CAD build for the part. Positions are in the model's coordinates, mm. Round coordinates to 2 decimals unless told otherwise and drop trailing zeros. Order: outer loops, then holes, each group sorted by start corner. A loop starts at its lowest first (then second) coordinate and runs counter-clockwise, first axis right, second up. Notation, with made-up numbers: (27, 26.25) -> (48, 26.25) arc R29 ccw to (48, 55.25) -> close; hole circle Ø9 at (84.25, -36). An arc over 180 degrees is marked (long way). Answer as CSV lines item,"result". Start each with the question number.
from build123d import *

# Parameters (mm, degrees)
SKETCH004_R          = 1.687519
PAD003_DEPTH         = 2
SKETCH003_R          = 1.746092
PAD002_DEPTH         = 2
FUSION001_ROLL_ANGLE = 90


with BuildPart() as base_and_horizontal_holder001:
    # Sketch004 → Pad003 (new body)
    with BuildSketch(Plane.XZ.offset(1.2525)):
        with BuildLine():
            Line((10.979984, 0), (69.999984, 0))
            Line((69.999984, 0), (69.999984, -21.282469))
            ThreePointArc((66.378106, -24.904346), (68.939161, -23.843523), (69.999984, -21.282469))
            Line((22.859289, -24.904346), (66.378106, -24.904346))
            ThreePointArc((10.979984, -13.025041), (14.459352, -21.424978), (22.859289, -24.904346))
            Line((10.979984, 0), (10.979984, -13.025041))
        make_face()
        with Locations((67.250754, -19)):
            Circle(SKETCH004_R, mode=Mode.SUBTRACT)
        with Locations((16.457754, -19)):
            Circle(SKETCH004_R, mode=Mode.SUBTRACT)
    extrude(amount=-PAD003_DEPTH)


with BuildPart() as obj1:
    # Sketch003 → Pad002 (new body)
    with BuildSketch(Plane(origin=(0, -0.167, -0.63), x_dir=(1, 0, 0), z_dir=(0, 0.5, 0.866025))):
        with BuildLine():
            Line((11.012519, -1.25328), (11.012519, 6.997142))
            ThreePointArc((13.001287, 8.992943), (11.59459, 8.405902), (11.012519, 6.997142))
            Line((13.001287, 8.992943), (15, 9))
            ThreePointArc((16.997615, 7.009425), (16.412099, 8.419465), (15, 9))
            Line((16.997615, 7.009425), (16.997615, 4))
            ThreePointArc((16.997615, 4), (17.290509, 3.292893), (17.997615, 3))
            Line((17.997615, 3), (62, 3))
            Line((62, 3), (62.401287, 3))
            ThreePointArc((62.401287, 3), (64.238855, 3.761145), (65, 5.598713))
            Line((65, 5.598713), (65, 6))
            Line((65, 6), (62, 10))
            ThreePointArc((65, 13), (62.87868, 12.12132), (62, 10))
            Line((65, 13), (67, 13))
            ThreePointArc((70, 10), (69.12132, 12.12132), (67, 13))
            Line((70, 10), (70, -1.25328))
            Line((11.012519, -1.25328), (70, -1.25328))
        make_face()
        with Locations((13.988471, 5.299093)):
            Circle(SKETCH003_R, mode=Mode.SUBTRACT)
        with Locations((66.082271, 10.342403)):
            Circle(SKETCH003_R, mode=Mode.SUBTRACT)
    extrude(amount=PAD002_DEPTH)

    # Fusion001: union base_and_horizontal_holder001
    add(base_and_horizontal_holder001.part)


with BuildPart() as obj1_1:
    # Fusion001 roll: moved
    add(obj1.part.rotate(Axis((0, 0, 0), (1, 0, 0)), FUSION001_ROLL_ANGLE))


with BuildPart() as obj1_2:
    # Fusion001 placement: moved
    add(obj1_1.part.moved(Location((-10.98, 2, 1.25))))


solid = obj1_2.part
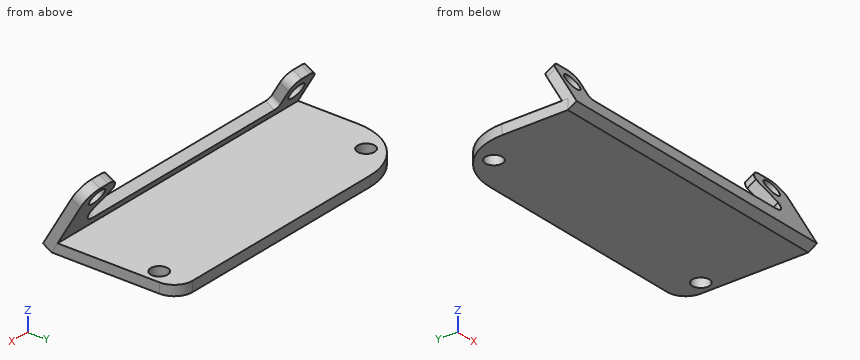
Item 1: Probe line 1 (X direction, y = 21, z = 0.85); line 2 (Z direction, x = 48.5, y = 5.25); line 3 (X direction, y = 5, z = 5.75). List the from-to ranges inside material, lowest first.
Item 2: Pin check, flat tips, straight feed: pin 1 (12.5 mm diameter, centred on x = 16.5, y = 16, fed in from +Z); pin 2 (2 mm diameter, centred on x = 5.48, y = 21, fed in from -Z); pin 3 (10 mm diameter, centred on x = 31, y = 9, fed in from +Z); pin 4 (1 mm diameter, centred on x = 35, z = 4, fed in from -Y). Stop position of each tip, or through.
Item 3: Band-saw the part on B-B, the plane y = 11.5. Give the cut face in (x, z), and give its area (3 significant figures).
Item 4: Band-saw the part on A-A, the plane y = 21. Give the cut face in (x, z).
Values:
1,line 1,"1.61 to 3.79, 7.17 to 54.58, 57.96 to 59.02"
1,line 2,"0 to 2"
1,line 3,"0.03 to 1.26, 4.75 to 6.02, 53.99 to 59.02"
2,pin 1,"z = 2"
2,pin 2,"through"
2,pin 3,"z = 3.76"
2,pin 4,"y = 1.72"
3,outline,"(0, 0) -> (59.02, 0) -> (59.02, 2) -> (0, 2) -> close"
3,area,"118 mm²"
4,outline,"(1.61, 0) -> (3.79, 0) -> (3.79, 2) -> (1.61, 2) -> close; (7.17, 0) -> (54.58, 0) -> (54.58, 2) -> (7.17, 2) -> close; (57.96, 0) -> (59.02, 0) -> (59.02, 2) -> (57.96, 2) -> close"
